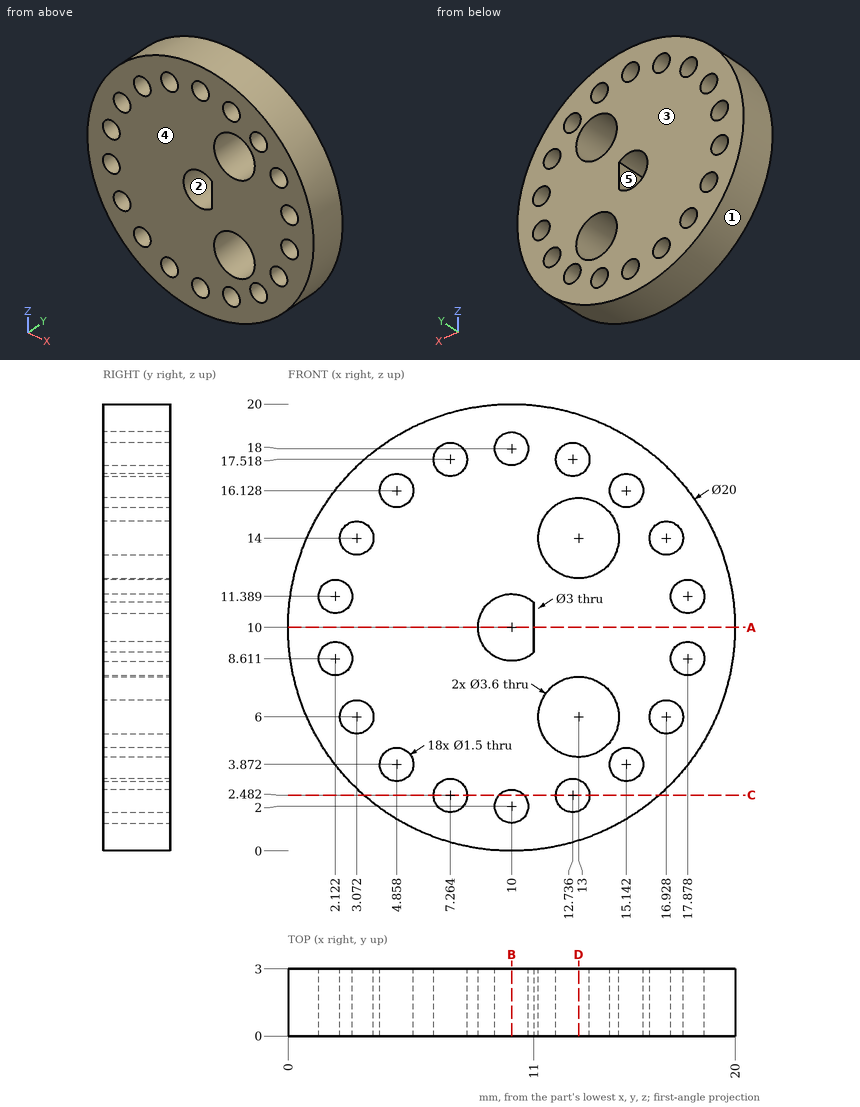
Design review of the part shown in the three views and the two pictorial views. Dimensions are in mm from the part's minimum x, y and z. A direction names the side the tool comes from. Round coordinates to 2 decimals unless told otherwise and drop trailing zeros. Write each loop counter-clockwise with the first axis right and the second up, starting at its lowest first coordinate (ties: lowest second). Pieces come first, ordered by that corner, then holes.
1) Take a section at D-D on x = 13. Give the boundary of the cut face in (y, z) (1 decimal).
Answer below:
outline: (0, 0.5) - (3, 0.5) - (3, 1.8) - (0, 1.8) - close; (0, 3.2) - (3, 3.2) - (3, 4.2) - (0, 4.2) - close; (0, 7.8) - (3, 7.8) - (3, 12.2) - (0, 12.2) - close; (0, 15.8) - (3, 15.8) - (3, 16.8) - (0, 16.8) - close; (0, 18.2) - (3, 18.2) - (3, 19.5) - (0, 19.5) - close
2) For line 1 along Z through (x, y) = (4.75, 2.8) (1 decimal); line 2 along X through (y, z) = (1.15, 14.25) (1 decimal); line 3 along X through (y, z) = (0.95, 6.5) (1 decimal), list the stretches that pass through material, from the lowest coordinate up.
Answer below:
line 1: z = 1.5 to 3.1, 4.6 to 15.4, 16.9 to 18.5
line 2: x = 0.9 to 2.4, 3.8 to 11.2, 14.8 to 16.2, 17.6 to 19.1
line 3: x = 0.6 to 2.5, 3.6 to 11.3, 14.7 to 16.4, 17.5 to 19.4
3) Take a section at A-A on z = 10. Give the boundary of the cut face in (x, y).
Answer below:
outline: (0, 0) - (8.5, 0) - (8.5, 3) - (0, 3) - close; (11, 0) - (20, 0) - (20, 3) - (11, 3) - close
4) Take a section at C-C on z = 2.5. Give the boundary of the cut face in (x, y) (1 decimal).
Answer below:
outline: (3.4, 0) - (6.5, 0) - (6.5, 3) - (3.4, 3) - close; (8, 0) - (9.4, 0) - (9.4, 3) - (8, 3) - close; (10.6, 0) - (12, 0) - (12, 3) - (10.6, 3) - close; (13.5, 0) - (16.6, 0) - (16.6, 3) - (13.5, 3) - close
5) Mouldability with a two-part tool opening along X and no side actions: class the marked faces 1, 2 and 3 as +X half, -X half, draft (parallel to the pull), parting line (faces both ways), or undercut.
Answer below:
face 1: parting line
face 2: undercut
face 3: draft
6) Machinability: for the marked faces 4 and 5, which of the approach directions +Z, -Z, +X, -X, +Y, -Y give a long, thin tool a straight path to every point of the face, cutting with its end or side? Answer none if there is none.
Answer below:
face 4: +Z, -Z, +X, -X, -Y
face 5: +Y, -Y
7) Take a section at B-B on x = 10. Give the boundary of the cut face in (y, z), then the cut area to 3 significant figures.
Answer below:
outline: (0, 0) - (3, 0) - (3, 1.25) - (0, 1.25) - close; (0, 2.75) - (3, 2.75) - (3, 8.5) - (0, 8.5) - close; (0, 11.5) - (3, 11.5) - (3, 17.25) - (0, 17.25) - close; (0, 18.75) - (3, 18.75) - (3, 20) - (0, 20) - close
area: 42.0 mm2
